Build history of the part. All positions in model axes, mm. A direction names the side the tool comes from. Coordinates: 2 decimals unless noted, no trailing zeros. Order: outer loops, then holes, each group sorted by start corner. A loop starts at its lowest first (then second) coordinate and runs counter-clockwise, first axis right, second up. Notation, with made-up numbers: M 8,87 L 55,87 A16 cw 55,107 Z; hole C 33.25,-18.5 d7. An arc over 180 degrees is marked long. Write item = value, one per line. Start each with the question number.
Q1. Band-saw the part on C-C on x = 22. Write the cut outline in (y, z).
Q2. Pin check, flat tips, straight feed: P1, Ø2.5, axis at x = -45, y = 9, coming from the +Z side; P2, Ø10, axis at y = 14, z = 17, coming from the -X side; P3, Ø4, axis at x = 33, z = 25, coming from the +Y side. Stop position of each tip, or through.
Q3. Band-saw the part on B-B on z = 6.5. Write the cut outline in (x, y), plus the area to 3 significant figures.
Q4. Pull direction Z, two halves, no side cores. Call faces 1 (the face through (-50, 1, 0)), 2 (the face through (-1, 1, 30)), 3 (the face through (-45, 7, 2)), 4 (the face through (18, 7, 20)): released by +Z, released by -Z, zero draft, split by the parting line, or undercut.
Q5. 3-axis set-ups, long thin cutter, end or side, ignore diameter. For faces 5 (the face through (-45, 7, -13)), 6 (the face through (27, 7, 24)), 7 (the face through (-1, 0, 0)), 8 (the face through (-49, 7, -5)), 9 (the face through (37, 7, 24)): which of +Z, -Z, +X, -X, +Y, -Y reach the whole face in a straight line?
Q6. Band-saw the part on D-D on y = 14.5. Write the cut outline in (x, z).
Q7. Drill centre lines: probe 1 along Z at (x, y) = (-42.5, 11.75); probe 2 along X at (y, z) = (4.5, 16.5); probe 3 along Y at (x, z) = (29, 9). Where is each one in solid material? Low to high.
Q8. Band-saw the part on A-A on y = 9.5. Write the cut outline in (x, z), plus the area to 3 significant figures.
```python
from build123d import *

# Parameters (mm, degrees)
SKETCH1_W           = 100
SKETCH1_H           = 60
BOSS_EXTRUDE1_DEPTH = 2
FILLET5_R           = 7
FILLET6_R           = 7
FILLET7_R           = 7
FILLET8_R           = 7
SKETCH2_W           = 8
SKETCH2_H           = 15
BOSS_EXTRUDE2_DEPTH = 10
SKETCH3_W           = 9
SKETCH3_H           = 15
BOSS_EXTRUDE3_DEPTH = 15
SKETCH4_W           = 10
SKETCH4_H           = 8
BOSS_EXTRUDE4_DEPTH = 10


with BuildPart() as part:
    # Sketch1 → Boss-Extrude1 (new body)
    with BuildSketch(Plane(origin=(0, 0, 0), x_dir=(1, 0, 0), z_dir=(0, 1, 0))):
        Rectangle(SKETCH1_W, SKETCH1_H)
    extrude(amount=BOSS_EXTRUDE1_DEPTH)

    # Fillet5
    fillet5_edges = [part.edges().sort_by_distance(p)[0] for p in [
        (50, 1, 30),
    ]]
    fillet(fillet5_edges, radius=FILLET5_R)

    # Fillet6
    fillet6_edges = [part.edges().sort_by_distance(p)[0] for p in [
        (50, 1, -30),
    ]]
    fillet(fillet6_edges, radius=FILLET6_R)

    # Fillet7
    fillet7_edges = [part.edges().sort_by_distance(p)[0] for p in [
        (-50, 1, -30),
    ]]
    fillet(fillet7_edges, radius=FILLET7_R)

    # Fillet8
    fillet8_edges = [part.edges().sort_by_distance(p)[0] for p in [
        (-50, 1, 30),
    ]]
    fillet(fillet8_edges, radius=FILLET8_R)

    # Sketch2 → Boss-Extrude2 (add)
    with BuildSketch(Plane(origin=(0, 2, 0), x_dir=(1, 0, 0), z_dir=(0, 1, 0))):
        with Locations((-45, 5.5)):
            Rectangle(SKETCH2_W, SKETCH2_H)
    extrude(amount=BOSS_EXTRUDE2_DEPTH)

    # Sketch3 → Boss-Extrude3 (add)
    with BuildSketch(Plane(origin=(0, 2, 0), x_dir=(1, 0, 0), z_dir=(0, 1, 0))):
        with Locations((-44.5, -11.5)):
            Rectangle(SKETCH3_W, SKETCH3_H)
    extrude(amount=BOSS_EXTRUDE3_DEPTH)

    # Sketch4 → Boss-Extrude4 (add)
    with BuildSketch(Plane(origin=(0, 2, 0), x_dir=(1, 0, 0), z_dir=(0, 1, 0))):
        with Locations((32, -24)):
            Rectangle(SKETCH4_W, SKETCH4_H)
        with Locations((18.5, -24)):
            Rectangle(SKETCH4_W, SKETCH4_H)
    extrude(amount=BOSS_EXTRUDE4_DEPTH)


solid = part.part
```
Recorded:
q1.outline = M 0,-30 L 2,-30 L 2,20 L 12,20 L 12,28 L 2,28 L 2,30 L 0,30 Z
q2.P1 = 19
q2.P2 = -49
q2.P3 = 12
q3.outline = M -50,0 L 50,0 L 50,2 L -40,2 L -40,17 L -49,17 L -49,2 L -50,2 Z
q3.area = 335 mm2
q4.face_1 = zero draft
q4.face_2 = released by +Z
q4.face_3 = undercut
q4.face_4 = released by -Z
q5.face_5 = -Z, +X, -X, +Y
q5.face_6 = +Z, -Z, +Y
q5.face_7 = +Z, -Z, +X, -X, -Y
q5.face_8 = +Z, -Z, -X, +Y
q5.face_9 = +Z, -Z, +X, +Y
q6.outline = M -49,4 L -40,4 L -40,19 L -49,19 Z
q7.probe_1 = -13 to 2, 4 to 19
q7.probe_2 = -49 to -40
q7.probe_3 = 0 to 2
q8.outline = M -49,-13 L -41,-13 L -41,2 L -49,2 Z; M -49,4 L -40,4 L -40,19 L -49,19 Z; M 13.5,20 L 23.5,20 L 23.5,28 L 13.5,28 Z; M 27,20 L 37,20 L 37,28 L 27,28 Z
q8.area = 415 mm2
